```python
from build123d import *

# Parameters (mm, degrees)
CROQUIS2_W              = 50.8
CROQUIS2_H              = 570.39
SALIENTE_EXTRUIR1_DEPTH = 6.31
CROQUIS3_W              = 50.8
CROQUIS3_H              = 6.31
SALIENTE_EXTRUIR2_DEPTH = 568.44
CROQUIS4_W              = 50.8
CROQUIS4_H              = 6.31
SALIENTE_EXTRUIR3_DEPTH = 1787.3
CROQUIS6_W              = 50.8
CROQUIS6_H              = 6.31
CROQUIS7_W              = 60
CROQUIS7_H              = 53.955
SALIENTE_EXTRUIR4_DEPTH = 6.31
CROQUIS8_W              = 60
CROQUIS8_H              = 6.31
CORTAR_EXTRUIR1_DEPTH   = 6.31
CROQUIS9_W              = 50.8
CROQUIS9_H              = 6.31


with BuildPart() as part:
    # Croquis2 → Saliente-Extruir1 (new body)
    with BuildSketch(Plane.XY):
        Rectangle(CROQUIS2_W, CROQUIS2_H)
    extrude(amount=SALIENTE_EXTRUIR1_DEPTH)

    # Croquis3 → Saliente-Extruir2 (add)
    with BuildSketch(Plane.XY.offset(6.31)):
        with Locations((0, -282.04)):
            Rectangle(CROQUIS3_W, CROQUIS3_H)
    extrude(amount=SALIENTE_EXTRUIR2_DEPTH)

    # Croquis4 → Saliente-Extruir3 (add)
    with BuildSketch(Plane(origin=(25.4, 0, 0), x_dir=(0, 0, -1), z_dir=(1, 0, 0))):
        with Locations((-549.35, -282.04)):
            Rectangle(CROQUIS4_W, CROQUIS4_H)
    extrude(amount=SALIENTE_EXTRUIR3_DEPTH)

    # Barrer1: sweep along a curve in space
    with BuildLine() as barrer1_path:
        Line((0, 282.04, 0), (0, 282.04, -204))
        Line((0, 282.04, -204), (0, 231.24, -204))
    # Croquis6 → Barrer1 (sweep)
    with BuildSketch(Plane(origin=(0, 0, 0), x_dir=(-1, 0, 0), z_dir=(0, 0, -1))):
        with Locations((0, 282.04)):
            Rectangle(CROQUIS6_W, CROQUIS6_H)
    sweep(path=barrer1_path.line, transition=Transition.RIGHT)

    # Croquis7 → Saliente-Extruir4 (add)
    with BuildSketch(Plane(origin=(0, 0, -207.155), x_dir=(-1, 0, 0), z_dir=(0, 0, -1))):
        with Locations((-55.4, 258.2175)):
            Rectangle(CROQUIS7_W, CROQUIS7_H)
    extrude(amount=-SALIENTE_EXTRUIR4_DEPTH)

    # Croquis8 → Cortar-Extruir1 (cut)
    with BuildSketch(Plane.XY.offset(-200.845)):
        with Locations((55.4, 282.04)):
            Rectangle(CROQUIS8_W, CROQUIS8_H)
    extrude(amount=-CORTAR_EXTRUIR1_DEPTH, mode=Mode.SUBTRACT)

    # Barrer2: sweep along a curve in space
    with BuildLine() as barrer2_path:
        Line((1787.3, -282.04, 574.75), (1787.3, -282.04, 601.16))
        Line((1787.3, -282.04, 601.16), (1787.3, -150.28, 601.16))
        Line((1787.3, -150.28, 601.16), (1787.3, -150.28, 1395.16))
    # Croquis9 → Barrer2 (sweep)
    with BuildSketch(Plane.XY.offset(574.75)):
        with Locations((1787.3, -282.04)):
            Rectangle(CROQUIS9_W, CROQUIS9_H)
    sweep(path=barrer2_path.line, transition=Transition.RIGHT)


solid = part.part
```
Here's how the part is built. I have some questions about the finished solid (model axes, mm). A direction names the side the tool comes from. Give positions to 0.01 mm unless a question says otherwise; leave off trailing zeros. Write each loop counter-clockwise with the first axis right and the second up, starting at its lowest first coordinate (ties: lowest second). Pieces come first, ordered by that corner, then holes. Notation, with made-up numbers: M -30.5,45.5 L -19.5,45.5 A13 ccw -19.5,68.5 Z; hole C -0.75,38.25 d8. An arc over 180 degrees is marked long. Put each result on its own line as item: value. Start each with the question number.
Item 1: Thinking about a two-plate mould opening in Z: for faces 1 (the flat face through (31, 255, -200.845)), 2 (the flat face through (0, 7, 6.31)), 3 (the flat face through (1812.7, -150, 962)), 4 (the flat face through (0, 278.885, -102)), which applies, +Z half, -Z half, draft (parallel to the pull), parting line (faces both ways), or undercut?
Item 2: I need wall thicknesses on L1, parallel to Y at x = 652, z = 554 (3 decimals). Which ranges of the line are inside material? Lowest first, please. Write a range as from..to.
Item 3: If we section it at B-B, the plane z = 1015: Write out the boundary of the cut face in (x, y) (3 decimals).
Item 4: If we section it at C-C, the plane x = 418.5: Write out the boundary of the cut face in (y, z) (3 decimals), then the cut area to 3 significant figures.
Item 5: On a 3-axis mill with a long thin cutter (end or side, diameter ignored), from which of +Z, -Z, +X, -X, +Y, -Y can I reach the whole of each face in a straight line? I mean faces 5 (the flat face through (1788, -212, 598.005)), 6 (the flat face through (1787, -218, 604.315)), 7 (the flat face through (685, -285.195, 527)). Say none if no direction works.
Item 6: If we section it at A-A, the plane y = -235: Write out the boundary of the cut face in (x, z) (3 decimals), then the cut area to 3 significant figures.
Item 7: Will these pins go through, and if not, where does the flat tip stop? pin 1 (5 mm diameter, centred on x = 43, z = -202.5, fed in from -Y); pin 2 (7 mm diameter, centred on x = 1044.5, y = -281.5, fed in from +Z); pin 3 (7 mm diameter, centred on y = 250.5, z = -203.5, fed in from +X).
Values:
1. face 1: undercut
1. face 2: +Z half
1. face 3: draft
1. face 4: undercut
2. L1: -285.195..-278.885
3. outline: M 1761.9,-153.435 L 1812.7,-153.435 L 1812.7,-147.125 L 1761.9,-147.125 Z
4. outline: M -285.195,523.95 L -278.885,523.95 L -278.885,574.75 L -285.195,574.75 Z
4. area: 321 mm²
5. face 5: -Z, +X, -X, +Y
5. face 6: +Z, +X, -X, -Y
5. face 7: +Z, -Z, +X, -X, -Y
6. outline: M -25.4,0 L 25.4,0 L 25.4,6.31 L -25.4,6.31 Z; M 1761.9,598.005 L 1812.7,598.005 L 1812.7,604.315 L 1761.9,604.315 Z
6. area: 641 mm²
7. pin 1: y = 231.24
7. pin 2: z = 574.75
7. pin 3: x = 85.4
